Design review of the part shown in the three views and the two pictorial views. Dimensions are in mm from the part's minimum x, y and z. Give positions to 0.01 mm unless a question says otherwise; leave off trailing zeros. Order: outer loops, then holes, each group sorted by start corner. A loop starts at its lowest first (then second) coordinate and runs counter-clockwise, first axis right, second up.
Item 1: For probe 1 along Y at (x, z) = (30, 5); probe 2 along X at (y, z) = (89.5, 9.75); probe 3 along Z at (x, y) = (21, 13), list the stretches that pass through material, from the lowest coordinate up.
Item 2: The part is to be moulded in two halves that separate along X. For the marked faces 1, 2 and 3, say which applies: released by +X, released by -X, zero draft, split by the parting line, or undercut.
Item 3: Consider section B-B (y = 15). Give the boundary of the cut face in (x, z), plus the area to 3 significant figures.
Item 4: For P1, Ø5, axis at x = 34.5, y = 65.5, coming from the +Z side; P2, Ø2, axis at x = 23.5, z = 12.5, coming from the +Y side, all flat-tipped, find the tip position at first contact; note any pin that passes through.
Item 5: Consider section C-C (z = 2.25). Give the boundary of the cut face in (x, y).
Item 6: Consider section D-D (y = 69). Give the boundary of the cut face in (x, z), plus the area to 3 significant figures.
Item 7: Consider section A-A (x = 30). Give the boundary of the cut face in (y, z).
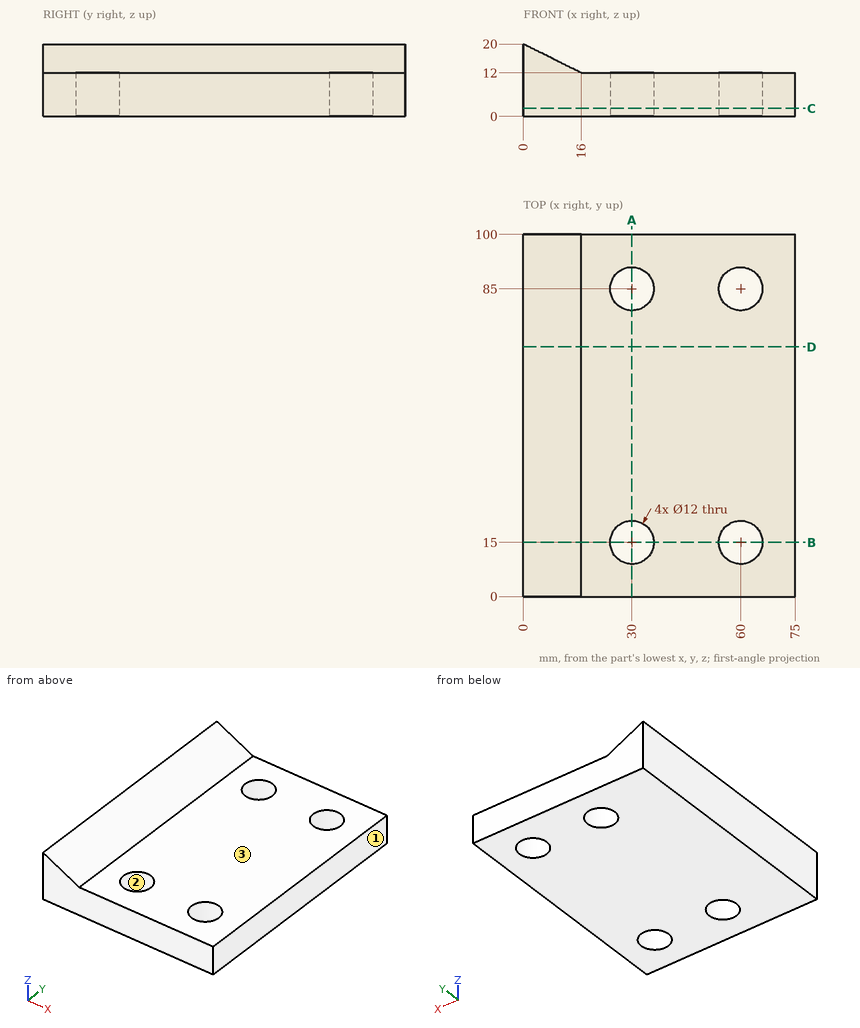
Resolved:
1. probe 1: y = 0 to 9, 21 to 79, 91 to 100
1. probe 2: x = 0 to 26.03, 33.97 to 56.03, 63.97 to 75
1. probe 3: z = 0 to 12
2. face 1: released by +X
2. face 2: undercut
2. face 3: zero draft
3. outline: (0, 0) - (24, 0) - (24, 12) - (16, 12) - (0, 20) - close; (36, 0) - (54, 0) - (54, 12) - (36, 12) - close; (66, 0) - (75, 0) - (75, 12) - (66, 12) - close
3. area: 676 mm2
4. P1: stops at z = 12
4. P2: stops at y = 100
5. outline: (0, 0) - (75, 0) - (75, 100) - (0, 100) - close; hole circle Ø12 at (30, 15); hole circle Ø12 at (30, 85); hole circle Ø12 at (60, 15); hole circle Ø12 at (60, 85)
6. outline: (0, 0) - (75, 0) - (75, 12) - (16, 12) - (0, 20) - close
6. area: 964 mm2
7. outline: (0, 0) - (9, 0) - (9, 12) - (0, 12) - close; (21, 0) - (79, 0) - (79, 12) - (21, 12) - close; (91, 0) - (100, 0) - (100, 12) - (91, 12) - close
